from build123d import *

# Parameters (mm, degrees)
SKETCH2_W           = 18
SKETCH2_H           = 1
BOSS_EXTRUDE2_DEPTH = 750
EDGE_FLANGE9_DEPTH  = 750
EDGE_FLANGE10_DEPTH = 750
SKETCH50_R          = 1.6
CUT_EXTRUDE1_DEPTH  = 10
SKETCH51_R          = 1.6
CUT_EXTRUDE2_DEPTH  = 10


# Sheet-metal steps are written as plain solids
with BuildPart() as part:
    # Sketch2 → Boss-Extrude2 (new body)
    with BuildSketch(Plane.XY):
        with Locations((-101.157096866, 298.73456983)):
            Rectangle(SKETCH2_W, SKETCH2_H)
    extrude(amount=BOSS_EXTRUDE2_DEPTH)

    # Edge-Flange9 section (across the edge) → Edge-Flange9 (add)
    with BuildSketch(Plane(origin=(-91.52201157, 299.23456983, 750), x_dir=(-0.8660254037844364, 0.5000000000000041, 0), z_dir=(0, 0, -1))):
        with BuildLine():
            Line((-1, 0.635085296), (-1, 30.422649731))
            Line((-1, 30.422649731), (0, 30.422649731))
            Line((0, 30.422649731), (0, 0.635085296))
            ThreePointArc((0, 0.635085296), (0.147372056, 0.085085296), (0.55, -0.317542648))
            Line((0.55, -0.317542648), (0.05, -1.183568052))
            ThreePointArc((0.05, -1.183568052), (-0.718653348, -0.414914704), (-1, 0.635085296))
        make_face()
    extrude(amount=EDGE_FLANGE9_DEPTH)

    # Edge-Flange10 section (across the edge) → Edge-Flange10 (add)
    with BuildSketch(Plane(origin=(-75.993144057, 326.131357347, 750), x_dir=(-0.8660254037844436, -0.49999999999999156, 0), z_dir=(0, 0, -1))):
        with BuildLine():
            Line((-1, 0.635085296), (-1, 18.64))
            Line((-1, 18.64), (0, 18.64))
            Line((0, 18.64), (0, 0.635085296))
            ThreePointArc((0, 0.635085296), (0.147372056, 0.085085296), (0.55, -0.317542648))
            Line((0.55, -0.317542648), (0.05, -1.183568052))
            ThreePointArc((0.05, -1.183568052), (-0.718653348, -0.414914704), (-1, 0.635085296))
        make_face()
    extrude(amount=EDGE_FLANGE10_DEPTH)

    # Sketch50 → Cut-Extrude1 (cut)
    with BuildSketch(Plane.XZ.offset(-298.23456983)):
        with Locations(Location((-106.227096866, 735, 0), (0, 0, 270))):
            Circle(SKETCH50_R)
        with Locations(Location((-106.227096866, 15, 0), (0, 0, 270))):
            Circle(SKETCH50_R)
        with Locations(Location((-106.227096866, 75, 0), (0, 0, 270))):
            Circle(SKETCH50_R)
        with Locations(Location((-106.227096866, 135, 0), (0, 0, 270))):
            Circle(SKETCH50_R)
        with Locations(Location((-106.227096866, 195, 0), (0, 0, 270))):
            Circle(SKETCH50_R)
        with Locations(Location((-106.227096866, 255, 0), (0, 0, 270))):
            Circle(SKETCH50_R)
        with Locations(Location((-106.227096866, 315, 0), (0, 0, 270))):
            Circle(SKETCH50_R)
        with Locations(Location((-106.227096866, 375, 0), (0, 0, 270))):
            Circle(SKETCH50_R)
        with Locations(Location((-106.227096866, 435, 0), (0, 0, 270))):
            Circle(SKETCH50_R)
        with Locations(Location((-106.227096866, 495, 0), (0, 0, 270))):
            Circle(SKETCH50_R)
        with Locations(Location((-106.227096866, 555, 0), (0, 0, 270))):
            Circle(SKETCH50_R)
        with Locations(Location((-106.227096866, 615, 0), (0, 0, 270))):
            Circle(SKETCH50_R)
        with Locations(Location((-106.227096866, 675, 0), (0, 0, 270))):
            Circle(SKETCH50_R)
    extrude(amount=-CUT_EXTRUDE1_DEPTH, mode=Mode.SUBTRACT)

    # Sketch51 → Cut-Extrude2 (cut)
    with BuildSketch(Plane(origin=(85.090187578, 49.126842704, 0), x_dir=(0, 0, -1), z_dir=(0.8660254037844434, 0.499999999999992, 0))):
        with Locations(Location((-735, 335.144612461, 0), (0, 0, 90))):
            Circle(SKETCH51_R)
        with Locations(Location((-15, 335.144612461, 0), (0, 0, 90))):
            Circle(SKETCH51_R)
        with Locations(Location((-75, 335.144612461, 0), (0, 0, 90))):
            Circle(SKETCH51_R)
        with Locations(Location((-135, 335.144612461, 0), (0, 0, 90))):
            Circle(SKETCH51_R)
        with Locations(Location((-195, 335.144612461, 0), (0, 0, 90))):
            Circle(SKETCH51_R)
        with Locations(Location((-255, 335.144612461, 0), (0, 0, 90))):
            Circle(SKETCH51_R)
        with Locations(Location((-315, 335.144612461, 0), (0, 0, 90))):
            Circle(SKETCH51_R)
        with Locations(Location((-375, 335.144612461, 0), (0, 0, 90))):
            Circle(SKETCH51_R)
        with Locations(Location((-435, 335.144612461, 0), (0, 0, 90))):
            Circle(SKETCH51_R)
        with Locations(Location((-495, 335.144612461, 0), (0, 0, 90))):
            Circle(SKETCH51_R)
        with Locations(Location((-555, 335.144612461, 0), (0, 0, 90))):
            Circle(SKETCH51_R)
        with Locations(Location((-615, 335.144612461, 0), (0, 0, 90))):
            Circle(SKETCH51_R)
        with Locations(Location((-675, 335.144612461, 0), (0, 0, 90))):
            Circle(SKETCH51_R)
    extrude(amount=-CUT_EXTRUDE2_DEPTH, mode=Mode.SUBTRACT)


solid = part.part
Geometry check sheet. Reference: the model listing, model coordinates, mm. A direction names the side the tool comes from. Give positions to 0.01 mm unless a question says otherwise; leave off trailing zeros. Write each loop counter-clockwise with the first axis right and the second up, starting at its lowest first coordinate (ties: lowest second). Pieces come first, ordered by that corner, then holes. Notation, with made-up numbers: (-29.5, -4) - (22.5, -4) arc R29 ccw to (22.5, 19) - close; hole circle Ø8 at (43.5, -28.5). An arc over 180 degrees is marked (long way). Put each result on its own line as item: value.
1. Set-up check for faces 1 (the flat face through (-82.996, 312.002, 380.25)), 2 (the flat face through (-101, 299.235, 370)), 3 (the flat face through (-83.653, 312.864, 380.25)): record each of +Z, -Z, +X, -X, +Y, -Y from which the full face is reachable in a straight line by a thin tool's end or side.
Ans:
face 1: +Z, -Z, +X, -Y
face 2: +Z, -Z, -X, +Y
face 3: +Z, -Z, -X
2. Sectioned sample at B-B, the plane y = 315. Enter the section's corners in (x, z).
Ans:
outline: (-82.42, 0) - (-81.27, 0) - (-81.27, 750) - (-82.42, 750) - close
3. Thickness scan on line 1 (X direction, y = 298.5, z = 555); line 2 (Y direction, x = -95, z = 304.5); line 3 (X direction, y = 298.95, z = 15). Record the ranges inside material, lowest first.
Ans:
line 1: x = -110.16 to -107.83, -104.63 to -91.14
line 2: y = 298.23 to 299.23
line 3: x = -110.16 to -107.83, -104.63 to -90.58
4. Sectioned sample at A-A, the plane z = 683. Enter the section's corners in (x, y).
Ans:
outline: (-110.16, 298.23) - (-92.16, 298.23) arc R2.1 ccw to (-90.34, 299.28) - (-75.44, 325.08) arc R2.1 ccw to (-75.44, 327.18) - (-84.45, 342.77) - (-85.31, 342.27) - (-76.31, 326.68) arc R1.1 cw to (-76.31, 325.58) - (-91.2, 299.78) arc R1.1 cw to (-92.16, 299.23) - (-110.16, 299.23) - close
5. Go/stop test with flat-tipped pins: pin 1 (4 mm diameter, centred on x = -106.23, z = 675, fed in from +Y); pin 2 (5 mm diameter, centred on x = -80, z = 220, fed in from -Y). Record where each tip stops, or that it passes through.
Ans:
pin 1: stops at y = 299.23
pin 2: stops at y = 312.86
